from build123d import *

# Parameters (mm, degrees)
F0_R     = 63.5
F1_DEPTH = 2.54
F2_R     = 4.09365
F3_DEPTH = 25.4
F4_DEPTH = 25.4
F5_W     = 19.05
F5_H     = 19.05
F6_DEPTH = 25.4


with BuildPart() as f1:
    # F0 (on Top) → F1 (new body)
    with BuildSketch(Plane.XY):
        Circle(F0_R)
    extrude(amount=F1_DEPTH)

    # F2 (on Top) → F3 (cut)
    with BuildSketch(Plane.XY):
        Circle(F2_R)
    extrude(amount=-F3_DEPTH, mode=Mode.SUBTRACT)

    # F2 (on Top) → F4 (cut)
    with BuildSketch(Plane.XY):
        Circle(F2_R)
    extrude(amount=F4_DEPTH, mode=Mode.SUBTRACT)

    # F5 (on Top) → F6 (cut)
    with BuildSketch(Plane.XY):
        with Locations((0, 24.230285)):
            Rectangle(F5_W, F5_H)
    extrude(amount=F6_DEPTH, mode=Mode.SUBTRACT)


solid = f1.part
Source: CAD feature listing. Evaluate the final solid. Frame: model axes, mm. Round coordinates to 2 decimals unless told otherwise and drop trailing zeros. Write each loop counter-clockwise with the first axis right and the second up, starting at its lowest first coordinate (ties: lowest second). Pieces come first, ordered by that corner, then holes. Notation, with made-up numbers: (77, 55.5) - (119, 55.5) arc R21 ccw to (119, 88.5) - close; hole circle Ø8 at (50, -14). An arc over 180 degrees is marked (long way). Use CSV: the item, a comma, the result in double quotes. Start each with the question number.
(1) Mould query, pull axis Y, two halves, no side actions, for faces 1 (the face through (-1, -13, 2.54)), 2 (the face through (-13.77, -61.99, 1.25)), 3 (the face through (-0.887, -3.996, 1.252)). Classes: pulls with the +Y half, pulls with the -Y half, needs draft (parallel to the pull), parting line crosses it, or undercut.
(2) Cut plane C-C, the plane z = 2.05. Return loops of the section in (x, y) (3 decimals).
(3) Cut plane A-A, the plane y = 0. Return loops of the section in (x, z).
(4) Material intervals for probe 1 along Y at (x, z) = (0, 1.75); probe 2 along Y at (x, z) = (-2.5, 1.4); probe 3 along X at (y, z) = (33.5, 0.85) (3 decimals), sorted ascending. Write a range as [from, to].
(5) Cut plane B-B, the plane x = 0. Return loops of the section in (y, z), and give its area (3 significant figures).
(6) Cut plane D-D, the plane x = -30. Return loops of the section in (y, z), and give its area (3 significant figures).
(7) First-contact query: pin 1 Ø1 at (y, z) = (-10, 1.5) entering from -X; pin 2 Ø0.8 at (x, z) = (-4.5, 1) entering from -Y; pin 3 Ø1.3 at (y, z) = (23.5, 1) entering from -X. Flat tips, straight axial feed; report the tip coordinate or a pass-through.
Geometry says:
1,face 1,"needs draft"
1,face 2,"parting line crosses it"
1,face 3,"undercut"
2,outline,"circle Ø127 at (0, 0); hole (-9.525, 14.705) - (9.525, 14.705) - (9.525, 33.755) - (-9.525, 33.755) - close; hole circle Ø8.187 at (0, 0)"
3,outline,"(-63.5, 0) - (-4.09, 0) - (-4.09, 2.54) - (-63.5, 2.54) - close; (4.09, 0) - (63.5, 0) - (63.5, 2.54) - (4.09, 2.54) - close"
4,probe 1,"[-63.5, -4.09], [4.09, 14.71], [33.76, 63.5]"
4,probe 2,"[-63.45, -3.24], [3.24, 14.71], [33.76, 63.45]"
4,probe 3,"[-53.944, -9.525], [9.525, 53.944]"
5,outline,"(-63.5, 0) - (-4.09, 0) - (-4.09, 2.54) - (-63.5, 2.54) - close; (4.09, 0) - (14.71, 0) - (14.71, 2.54) - (4.09, 2.54) - close; (33.76, 0) - (63.5, 0) - (63.5, 2.54) - (33.76, 2.54) - close"
5,area,"253 mm²"
6,outline,"(-55.97, 0) - (55.97, 0) - (55.97, 2.54) - (-55.97, 2.54) - close"
6,area,"284 mm²"
7,pin 1,"x = -62.79"
7,pin 2,"y = -63.37"
7,pin 3,"x = -59.25"
